```python
from build123d import *

# Parameters (mm, degrees)
SKETCH_1_W          = 20
SKETCH_1_H          = 40
EXTRUDE_1_DEPTH     = 8
SKETCH_2_R          = 1.5
CUT_EXTRUDE_1_DEPTH = 46.431266766
SKETCH_3_W          = 9
SKETCH_3_H          = 40
CUT_EXTRUDE_2_DEPTH = 4


with BuildPart() as part:
    # 草图1 → 凸台-拉伸1 (new body)
    with BuildSketch(Plane(origin=(0, 0, 0), x_dir=(1, 0, 0), z_dir=(0, 1, 0))):
        with Locations((10, -20)):
            Rectangle(SKETCH_1_W, SKETCH_1_H)
    extrude(amount=EXTRUDE_1_DEPTH)

    # 草图2 → 切除-拉伸1 (cut, through all)
    with BuildSketch(Plane(origin=(0, 8, 0), x_dir=(1, 0, 0), z_dir=(0, 1, 0))):
        with Locations(Location((2.5, -28, 0), (0, 0, 270))):
            Circle(SKETCH_2_R)
        with Locations(Location((17.5, -28, 0), (0, 0, 270))):
            Circle(SKETCH_2_R)
        with Locations(Location((17.5, -12, 0), (0, 0, 270))):
            Circle(SKETCH_2_R)
        with Locations(Location((2.5, -12, 0), (0, 0, 270))):
            Circle(SKETCH_2_R)
    extrude(amount=-CUT_EXTRUDE_1_DEPTH, mode=Mode.SUBTRACT)

    # 草图3 → 切除-拉伸2 (cut)
    with BuildSketch(Plane(origin=(0, 8, 0), x_dir=(1, 0, 0), z_dir=(0, 1, 0))):
        with Locations((10, -20)):
            Rectangle(SKETCH_3_W, SKETCH_3_H)
    extrude(amount=-CUT_EXTRUDE_2_DEPTH, mode=Mode.SUBTRACT)


solid = part.part
```
Geometry check sheet. Reference: the model listing, model coordinates, mm. A direction names the side the tool comes from. Give positions to 0.01 mm unless a question says otherwise; leave off trailing zeros. Order: outer loops, then holes, each group sorted by start corner. A loop starts at its lowest first (then second) coordinate and runs counter-clockwise, first axis right, second up.
1. Release check for a two-part mould opening along Z. For faces 1 (the face through (2.57, 4.06, 26.5)), 2 (the face through (17, 8, 20)), 3 (the face through (10, 3, 40)) record: pulls with the +Z half, pulls with the -Z half, needs draft (parallel to the pull), parting line crosses it, or undercut.
2. Section check A-A, the plane y = 5. Enter the section's corners in (x, z).
3. Thickness scan on L1, parallel to X at y = 2.75, z = 12; L2, parallel to X at y = 6.25, z = 28; L3, parallel to X at y = 6.5, z = 9.5. Record the ranges inside material, lowest first.
4. Access from +Z, -Z, +X, -X, +Y, -Y to the whole of each face (thin tool, end or side, straight path). Record for faces 4 (the face through (18.51, 4.06, 10.89)), 5 (the face through (10, 4, 20)).
5. Section check B-B, the plane x = 2.5. Enter the section's corners in (y, z), and give its area (3 significant figures).
6. Gauge pin test, flat end, axial feed: pin 1 Ø4.5 at (x, z) = (11, 20) entering from +Y. Record the tip position at first contact, or that the pin passes through.
7. Section check D-D, the plane y = 3. Enter the section's corners in (x, z).
8. Section check C-C, the plane z = 12. Enter the section's corners in (x, y).
Values follow:
1. face 1: undercut
1. face 2: needs draft
1. face 3: pulls with the +Z half
2. outline: (0, 0) - (5.5, 0) - (5.5, 40) - (0, 40) - close; (14.5, 0) - (20, 0) - (20, 40) - (14.5, 40) - close; hole circle Ø3 at (2.5, 12); hole circle Ø3 at (2.5, 28); hole circle Ø3 at (17.5, 12); hole circle Ø3 at (17.5, 28)
3. L1: x = 0 to 1, 4 to 16, 19 to 20
3. L2: x = 0 to 1, 4 to 5.5, 14.5 to 16, 19 to 20
3. L3: x = 0 to 5.5, 14.5 to 20
4. face 4: +Y, -Y
4. face 5: +Z, -Z, +Y
5. outline: (0, 0) - (8, 0) - (8, 10.5) - (0, 10.5) - close; (0, 13.5) - (8, 13.5) - (8, 26.5) - (0, 26.5) - close; (0, 29.5) - (8, 29.5) - (8, 40) - (0, 40) - close
5. area: 272 mm2
6. pin 1: stops at y = 4
7. outline: (0, 0) - (20, 0) - (20, 40) - (0, 40) - close; hole circle Ø3 at (2.5, 12); hole circle Ø3 at (2.5, 28); hole circle Ø3 at (17.5, 12); hole circle Ø3 at (17.5, 28)
8. outline: (0, 0) - (1, 0) - (1, 8) - (0, 8) - close; (4, 0) - (16, 0) - (16, 8) - (14.5, 8) - (14.5, 4) - (5.5, 4) - (5.5, 8) - (4, 8) - close; (19, 0) - (20, 0) - (20, 8) - (19, 8) - close
